```python
from build123d import *
from build123d.topology import SkipClean

# Parameters (mm, degrees)
SKETCH_1_W           = 80
SKETCH_1_H           = 54
SKETCH_1_W_2         = 76
SKETCH_1_H_2         = 50
EXTRUDE_1_DEPTH      = 24
SKETCH_2_W           = 80
SKETCH_2_H           = 54
EXTRUDE_1_2_DEPTH    = 2
SKETCH_3_R           = 2.8
SKETCH_3_R_2         = 1.45
EXTRUDE_4_DEPTH      = 3
SKETCH_4_W           = 16
SKETCH_4_H           = 10
SKETCH_4_W_2         = 12
SKETCH_4_H_2         = 9
CUT_EXTRUDE_1_DEPTH  = 2
SKETCH_6_W           = 10
SKETCH_6_H           = 12.5
CUT_EXTRUDE_2_DEPTH  = 2
CUT_EXTRUDE_START    = -2
SKETCH_7_R           = 1.45
CUT_EXTRUDE_3_DEPTH  = 2
SKETCH_8_W           = 81
SKETCH_8_H           = 5.5
CUT_EXTRUDE_4_DEPTH  = 2
EXTRUDE_5_DEPTH      = 2
EXTRUDE_6_DEPTH      = 3.5
SKETCH_11_W          = 45
SKETCH_11_H          = 22
CUT_EXTRUDE_5_DEPTH  = 8
EXTRUDE_7_DEPTH      = 6
SKETCH_13_W          = 53
SKETCH_13_H          = 22
EXTRUDE_8_DEPTH      = 2
SKETCH_14_R          = 2.3
SKETCH_14_R_2        = 1.45
SKETCH_14_R_3        = 0.95
EXTRUDE_9_DEPTH      = 2
SKETCH_15_R          = 1.45
CUT_EXTRUDE_6_DEPTH  = 2
EXTRUDE_10_DEPTH     = 2
CUT_EXTRUDE_7_DEPTH  = 2
EXTRUDE_11_DEPTH     = 1
CUT_EXTRUDE_START_2  = -1
CUT_EXTRUDE_8_DEPTH  = 1
SKETCH_20_R          = 3
CUT_EXTRUDE_9_DEPTH  = 1
SKETCH_21_R          = 3
CUT_EXTRUDE_10_DEPTH = 1


with BuildPart() as part:
    # Эскиз1 → Extrude 1 (new body)
    with BuildSketch(Plane.XY):
        Rectangle(SKETCH_1_W, SKETCH_1_H)
        Rectangle(SKETCH_1_W_2, SKETCH_1_H_2, mode=Mode.SUBTRACT)
    extrude(amount=EXTRUDE_1_DEPTH)

    # Эскиз2 → Extrude 1 2 (add)
    with BuildSketch(Plane(origin=(0, 0, 0), x_dir=(-1, 0, 0), z_dir=(0, 0, -1))):
        Rectangle(SKETCH_2_W, SKETCH_2_H)
    extrude(amount=EXTRUDE_1_2_DEPTH)

    # Эскиз3 → Бобышка-Вытянуть4 (add)
    # profile 1 of 4: a face of its own
    with BuildSketch(Plane.XY):
        with Locations((35, 19.75)):
            Circle(SKETCH_3_R)
        with Locations((35, 19.75)):
            Circle(SKETCH_3_R_2, mode=Mode.SUBTRACT)
    # profile 2 of 4: a face of its own
    with BuildSketch(Plane.XY):
        with Locations((35, -14.25)):
            Circle(SKETCH_3_R)
        with Locations((35, -14.25)):
            Circle(SKETCH_3_R_2, mode=Mode.SUBTRACT)
    # profile 3 of 4: a face of its own
    with BuildSketch(Plane.XY):
        with Locations((-35, -14.25)):
            Circle(SKETCH_3_R)
        with Locations((-35, -14.25)):
            Circle(SKETCH_3_R_2, mode=Mode.SUBTRACT)
    # profile 4 of 4: a face of its own
    with BuildSketch(Plane.XY):
        with Locations((-35, 19.75)):
            Circle(SKETCH_3_R)
        with Locations((-35, 19.75)):
            Circle(SKETCH_3_R_2, mode=Mode.SUBTRACT)
    extrude(amount=EXTRUDE_4_DEPTH)

    # Эскиз4 → Вырез-Вытянуть1 (cut)
    with BuildSketch(Plane.XZ.offset(27)):
        with Locations((23.5, 8)):
            Rectangle(SKETCH_4_W, SKETCH_4_H)
        with Locations((5, 19.5)):
            Rectangle(SKETCH_4_W_2, SKETCH_4_H_2)
    extrude(amount=-CUT_EXTRUDE_1_DEPTH, mode=Mode.SUBTRACT)

    # Эскиз6 → Вырез-Вытянуть2 (cut)
    with BuildSketch(Plane(origin=(0, 27, 0), x_dir=(1, 0, 0), z_dir=(0, 1, 0))):
        with Locations((-26.5, -10.25)):
            Rectangle(SKETCH_6_W, SKETCH_6_H)
    extrude(amount=-CUT_EXTRUDE_2_DEPTH, mode=Mode.SUBTRACT)

    # Эскиз7 → Вырез-Вытянуть3 (cut)
    with BuildSketch(Plane.XY.offset(CUT_EXTRUDE_START)):
        with Locations((-35, 19.75)):
            Circle(SKETCH_7_R)
        with Locations((-35, -14.25)):
            Circle(SKETCH_7_R)
        with Locations((35, 19.75)):
            Circle(SKETCH_7_R)
        with Locations((35, -14.25)):
            Circle(SKETCH_7_R)
    extrude(amount=CUT_EXTRUDE_3_DEPTH, mode=Mode.SUBTRACT)

    # Эскиз8 → Вырез-Вытянуть4 (cut)
    with BuildSketch(Plane(origin=(0, 27, 0), x_dir=(1, 0, 0), z_dir=(0, 1, 0))):
        with Locations((0, -21.25)):
            Rectangle(SKETCH_8_W, SKETCH_8_H)
    extrude(amount=-CUT_EXTRUDE_4_DEPTH, mode=Mode.SUBTRACT)

    # Эскиз9 → Бобышка-Вытянуть5 (add)
    with BuildSketch(Plane.XY.offset(18.5)):
        Polygon((42.5, 25), (42.5, 63), (-42.5, 63), (-42.5, 25), (-42.5, 24.5), (-40, 24.5), (-40, 25), (40, 25), (40, 24.5), (42.5, 24.5), align=None)
    extrude(amount=EXTRUDE_5_DEPTH)

    # Эскиз10 → Бобышка-Вытянуть6 (add)
    with BuildSketch(Plane.XY.offset(20.5)):
        Polygon((40.5, 25), (40.5, 61), (-40.5, 61), (-40.5, 25), (-40, 25), (-40, 24.5), (-42.5, 24.5), (-42.5, 25), (-42.5, 63), (42.5, 63), (42.5, 25), (42.5, 24.5), (40, 24.5), (40, 25), align=None)
    extrude(amount=EXTRUDE_6_DEPTH)

    # Эскиз11 → Вырез-Вытянуть5 (cut)
    with BuildSketch(Plane.XY.offset(20.5)):
        with Locations((13, 36)):
            Rectangle(SKETCH_11_W, SKETCH_11_H)
    extrude(amount=-CUT_EXTRUDE_5_DEPTH, mode=Mode.SUBTRACT)

    # Эскиз12 → Бобышка-Вытянуть7 (add)
    with BuildSketch(Plane(origin=(0, 0, 18.5), x_dir=(-1, 0, 0), z_dir=(0, 0, -1))):
        Polygon((9.5, 27), (15.5, 27), (15.5, 49), (-37.5, 49), (-37.5, 27), (-35.5, 27), (-35.5, 47), (9.5, 47), align=None)
    extrude(amount=EXTRUDE_7_DEPTH)

    # Эскиз13 → Бобышка-Вытянуть8 (add)
    with BuildSketch(Plane(origin=(0, 0, 12.5), x_dir=(-1, 0, 0), z_dir=(0, 0, -1))):
        with Locations((-11, 38)):
            Rectangle(SKETCH_13_W, SKETCH_13_H)
    extrude(amount=EXTRUDE_8_DEPTH)

    # Эскиз14 → Бобышка-Вытянуть9 (add)
    # profile 1 of 4: a face of its own
    with BuildSketch(Plane.XY.offset(20.5)):
        with Locations((37.75, 58.5)):
            Circle(SKETCH_14_R)
        with Locations((37.75, 58.5)):
            Circle(SKETCH_14_R_2, mode=Mode.SUBTRACT)
    # profile 2 of 4: a face of its own
    with BuildSketch(Plane.XY.offset(20.5)):
        with Locations(Location((37.75, 27.5, 0), (0, 0, 191.968745555))):
            Circle(SKETCH_14_R)
        with Locations((37.75, 27.5)):
            Circle(SKETCH_14_R_3, mode=Mode.SUBTRACT)
    # profile 3 of 4: a face of its own
    with BuildSketch(Plane.XY.offset(20.5)):
        with Locations((-37.75, 58.5)):
            Circle(SKETCH_14_R)
        with Locations((-37.75, 58.5)):
            Circle(SKETCH_14_R_2, mode=Mode.SUBTRACT)
    # profile 4 of 4: a face of its own
    with BuildSketch(Plane.XY.offset(20.5)):
        with Locations((-37.75, 27.5)):
            Circle(SKETCH_14_R)
        with Locations((-37.75, 27.5)):
            Circle(SKETCH_14_R_3, mode=Mode.SUBTRACT)
    extrude(amount=EXTRUDE_9_DEPTH)

    # Эскиз15 → Вырез-Вытянуть6 (cut)
    with BuildSketch(Plane.XY.offset(20.5).offset(CUT_EXTRUDE_START)):
        with Locations((-37.75, 58.5)):
            Circle(SKETCH_15_R)
        with Locations((37.75, 58.5)):
            Circle(SKETCH_15_R)
    extrude(amount=CUT_EXTRUDE_6_DEPTH, mode=Mode.SUBTRACT)

    # Эскиз16 → Бобышка-Вытянуть10 (add)
    # profile 1 of 2: a face of its own
    with BuildSketch(Plane.XY):
        with BuildLine():
            Line((-14, 10), (-14, 0))
            ThreePointArc((-14, 0), (-20, -6), (-26, 0))
            Line((-26, 0), (-26, 10))
            ThreePointArc((-26, 10), (-20, 16), (-14, 10))
        make_face()
        with BuildLine():
            Line((-25, 10), (-25, 0))
            ThreePointArc((-25, 0), (-20, -5), (-15, 0))
            Line((-15, 0), (-15, 10))
            ThreePointArc((-15, 10), (-20, 15), (-25, 10))
        make_face(mode=Mode.SUBTRACT)
    # profile 2 of 2: a face of its own
    with BuildSketch(Plane.XY):
        with BuildLine():
            Line((26, 10), (26, 0))
            ThreePointArc((26, 0), (20, -6), (14, 0))
            Line((14, 0), (14, 10))
            ThreePointArc((14, 10), (20, 16), (26, 10))
        make_face()
        with BuildLine():
            Line((15, 10), (15, 0))
            ThreePointArc((15, 0), (20, -5), (25, 0))
            Line((25, 0), (25, 10))
            ThreePointArc((25, 10), (20, 15), (15, 10))
        make_face(mode=Mode.SUBTRACT)
    extrude(amount=EXTRUDE_10_DEPTH)

    # Эскиз17 → Вырез-Вытянуть7 (cut)
    with SkipClean():  # the faces are left unmerged after this step: merging them gives an invalid solid
        with BuildSketch(Plane.XY.offset(CUT_EXTRUDE_START)):
            with BuildLine():
                Line((-18, 2), (-18, 3.195989192))
                ThreePointArc((-18, 3.195989192), (-17.651483717, 4.828982354), (-16.666666667, 6.177413162))
                ThreePointArc((-16.666666667, 6.177413162), (-20, 14.904193125), (-23.333333333, 6.177413162))
                ThreePointArc((-23.333333333, 6.177413162), (-22.348516283, 4.828982354), (-22, 3.195989192))
                Line((-22, 3.195989192), (-22, 2))
                Line((-22, 2), (-22, 0))
                ThreePointArc((-22, 0), (-20, -2), (-18, 0))
                Line((-18, 0), (-18, 2))
            make_face()
            with BuildLine():
                Line((18, 0), (18, 2))
                Line((18, 2), (18, 3.291796068))
                ThreePointArc((18, 3.291796068), (17.651483717, 4.924789229), (16.666666667, 6.273220038))
                ThreePointArc((16.666666667, 6.273220038), (20, 15), (23.333333333, 6.273220038))
                ThreePointArc((23.333333333, 6.273220038), (22.348516283, 4.924789229), (22, 3.291796068))
                Line((22, 3.291796068), (22, 2))
                Line((22, 2), (22, 0))
                ThreePointArc((22, 0), (20, -2), (18, 0))
            make_face()
        extrude(amount=CUT_EXTRUDE_7_DEPTH, mode=Mode.SUBTRACT)

    # Эскиз18 → Бобышка-Вытянуть11 (add)
    with SkipClean():  # the faces are left unmerged after this step: merging them gives an invalid solid
        with BuildSketch(Plane.XY.offset(2)):
            with BuildLine():
                Line((22, 0), (22, 3))
                Line((22, 3), (26, 3))
                Line((26, 3), (26, 0))
                ThreePointArc((26, 0), (20, -6), (14, 0))
                Line((14, 0), (14, 3))
                Line((14, 3), (15, 3))
                Line((15, 3), (18, 3))
                Line((18, 3), (18, 0))
                ThreePointArc((18, 0), (20, -2), (22, 0))
            make_face()
            with BuildLine():
                Line((-14, 0), (-14, 3))
                Line((-14, 3), (-17, 3))
                Line((-17, 3), (-17, 0))
                ThreePointArc((-17, 0), (-20, -3), (-23, 0))
                Line((-23, 0), (-23, 3))
                Line((-23, 3), (-26, 3))
                Line((-26, 3), (-26, 0))
                ThreePointArc((-26, 0), (-20, -6), (-14, 0))
            make_face()
        extrude(amount=EXTRUDE_11_DEPTH)

    # Эскиз19 → Вырез-Вытянуть8 (cut)
    with BuildSketch(Plane.XY.offset(CUT_EXTRUDE_START_2)):
        with BuildLine():
            Line((-25, 0), (-25, 10))
            ThreePointArc((-25, 10), (-20, 15), (-15, 10))
            Line((-15, 10), (-15, 0))
            ThreePointArc((-15, 0), (-20, -5), (-25, 0))
        make_face()
        with BuildLine():
            Line((25, 10), (25, 0))
            ThreePointArc((25, 0), (20, -5), (15, 0))
            Line((15, 0), (15, 10))
            ThreePointArc((15, 10), (20, 15), (25, 10))
        make_face()
    extrude(amount=CUT_EXTRUDE_8_DEPTH, mode=Mode.SUBTRACT)

    # Эскиз20 → Вырез-Вытянуть9 (cut)
    with BuildSketch(Plane(origin=(0, 0, -2), x_dir=(-1, 0, 0), z_dir=(0, 0, -1))):
        with Locations((35, -14.25)):
            Circle(SKETCH_20_R)
        with Locations((35, 19.75)):
            Circle(SKETCH_20_R)
        with Locations((-35, -14.25)):
            Circle(SKETCH_20_R)
        with Locations((-35, 19.75)):
            Circle(SKETCH_20_R)
    extrude(amount=-CUT_EXTRUDE_9_DEPTH, mode=Mode.SUBTRACT)

    # Эскиз21 → Вырез-Вытянуть10 (cut)
    with BuildSketch(Plane(origin=(0, 0, 18.5), x_dir=(-1, 0, 0), z_dir=(0, 0, -1))):
        with Locations((37.75, 58.5)):
            Circle(SKETCH_21_R)
        with Locations((-37.75, 58.5)):
            Circle(SKETCH_21_R)
    extrude(amount=-CUT_EXTRUDE_10_DEPTH, mode=Mode.SUBTRACT)


solid = part.part
```
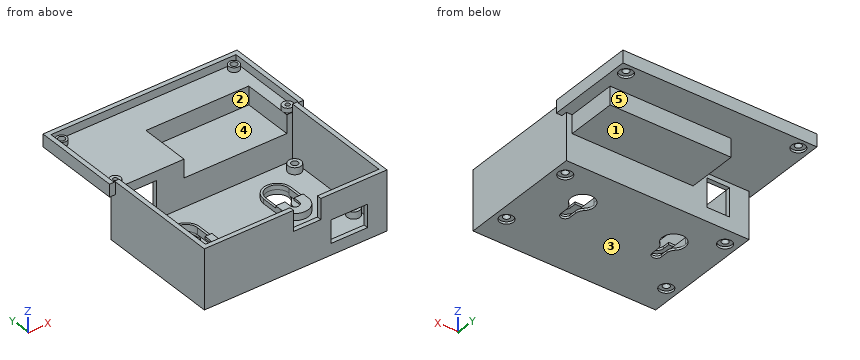
Check sheet for the modelled part. Datum: model origin and axes. Units: mm. Face numbers are marked on the shaded views. A direction names the side the tool comes from. Give positions to 0.01 mm unless a question says otherwise; leave off trailing zeros. Write each loop counter-clockwise with the first axis right and the second up, starting at its lowest first coordinate (ties: lowest second). Pieces come first, ordered by that corner, then holes.
Item 1: Cross-section at B-B (z = 9). Enter the section's corners in (x, y).
Item 2: Access from +Z, -Z, +X, -X, +Y, -Y to the whole of each face (thin tool, end or side, straight path). Record for the marked faces 1, 2 and 3.
Item 3: Cross-section at C-C (x = -5). Enter the section's corners in (y, z).
Item 4: Draft check along X on the marked faces 4 and 5. Enter one of: released by +X, released by -X, zero draft, split by the parting line, or undercut.
Item 5: Cross-section at D-D (y = 39). Enter the section's corners in (x, z), and give its area (3 significant figures).
Item 6: Scan lines: L1, parallel to Y at x = -35, z = 0.7; L2, parallel to Y at x = 37.75, z = 21.5; L3, parallel to Y at x = -35, z = -1.7. Record each from-to range of solid material in increasing order.
Item 7: Gauge pin test, flat ends, axial feed: pin 1 (13 mm diameter, centred on y = 12, z = 6, fed in from -X); pin 2 (0.6 mm diameter, centred on y = -26, z = 9, fed in from +X); pin 3 (4 mm diameter, centred on x = -25, y = 51, fed in from +Z). Record the tip position at first contact, or that the pin passes through.
Item 8: Cross-section at A-A (y = -14.25). Count the separate pieces of the cut face and the enclosed holes in it, and give its area (3 significant figures).
Report:
1. outline: (-40, -27) - (15.5, -27) - (15.5, -25) - (-38, -25) - (-38, 25) - (-31.5, 25) - (-31.5, 27) - (-40, 27) - close; (-21.5, 25) - (38, 25) - (38, -25) - (31.5, -25) - (31.5, -27) - (40, -27) - (40, 27) - (-21.5, 27) - close
2. face 1: -Z, +X, -X, +Y
2. face 2: +Z
2. face 3: -Z, +X, -X, +Y, -Y
3. outline: (-27, -2) - (27, -2) - (27, 10.5) - (49, 10.5) - (49, 18.5) - (63, 18.5) - (63, 24) - (61, 24) - (61, 20.5) - (47, 20.5) - (47, 12.5) - (25, 12.5) - (25, 0) - (-25, 0) - (-25, 24) - (-27, 24) - close
4. face 4: undercut
4. face 5: zero draft
5. outline: (-42.5, 18.5) - (-15.5, 18.5) - (-15.5, 10.5) - (37.5, 10.5) - (37.5, 18.5) - (42.5, 18.5) - (42.5, 24) - (40.5, 24) - (40.5, 20.5) - (35.5, 20.5) - (35.5, 12.5) - (-9.5, 12.5) - (-9.5, 20.5) - (-40.5, 20.5) - (-40.5, 24) - (-42.5, 24) - close
5. area: 248 mm2
6. L1: y = -27 to -25, -17.05 to -15.7, -12.8 to -11.45, 16.95 to 18.3, 21.2 to 22.55, 25 to 27
6. L2: y = -27 to -25, 25.2 to 26.55, 28.45 to 29.8, 56.2 to 57.05, 59.95 to 60.8, 61 to 63
6. L3: y = -27 to -17.25, -11.25 to 16.75, 22.75 to 27
7. pin 1: stops at x = -40
7. pin 2: stops at x = 40
7. pin 3: stops at z = 20.5
8. separate pieces: 3
8. enclosed holes: 0
8. area: 254 mm2
